from build123d import *

# Parameters (mm, degrees)
F0_W     = 152.4
F0_H     = 50.8
F1_DEPTH = 76.2
F3_DEPTH = 76.201
F5_DEPTH = 152.401


with BuildPart() as f1:
    # F0 (on Front) → F1 (new body)
    with BuildSketch(Plane.XZ):
        with Locations((8.127087, 3.526762)):
            Rectangle(F0_W, F0_H)
    extrude(amount=F1_DEPTH)

    # F2 (on face) → F3 (cut, through all)
    with BuildSketch(Plane.XZ.offset(76.2)):
        Polygon((-40.834155, -12.95126), (-29.972913, -21.873238), (53.436877, -21.873238), (60.765845, -12.95126), align=None)
    extrude(amount=-F3_DEPTH, mode=Mode.SUBTRACT)

    # F4 (on face) → F5 (cut, through all)
    with BuildSketch(Plane.YZ.offset(84.327087)):
        Polygon((-25.4, 28.926762), (-50.8, 28.926762), (-50.8, 16.226762), (-63.5, 16.226762), (-63.5, 3.526762), (-12.7, 3.526762), (-12.7, 16.226762), (-25.4, 16.226762), align=None)
    extrude(amount=-F5_DEPTH, mode=Mode.SUBTRACT)


solid = f1.part
Here's how the part is built. I have some questions about the finished solid (model axes, mm). A direction names the side the tool comes from. Round coordinates to 2 decimals unless told otherwise and drop trailing zeros. Write each loop counter-clockwise with the first axis right and the second up, starting at its lowest first coordinate (ties: lowest second). Pieces come first, ordered by that corner, then holes. Notation, with made-up numbers: (5.5, 19.5) -> (30.5, 19.5) arc R20 cw to (30.5, 27.5) -> close; hole circle Ø8 at (30, -9.75). An arc over 180 degrees is marked (long way). One line per item, written item: value.
1) If I drill on line 1 (Z direction, x = 34.5, y = -20); line 2 (Y direction, x = -54, z = 10.5); line 3 (Y direction, x = -46.5, z = 18.5), over which ranges is the centre line in solid material (lowest first)? Write a range as [from, to].
Filled sheet:
line 1: z = [-12.95, 3.53], [16.23, 28.93]
line 2: y = [-76.2, -63.5], [-12.7, 0]
line 3: y = [-76.2, -50.8], [-25.4, 0]
2) Suppose I cut it at B-B on y = -40.5. List the corners of the cut face in (x, z) for me, plus the area to 3 significant figures.
Filled sheet:
outline: (-68.07, -21.87) -> (-29.97, -21.87) -> (-40.83, -12.95) -> (60.77, -12.95) -> (53.44, -21.87) -> (84.33, -21.87) -> (84.33, 3.53) -> (-68.07, 3.53) -> close
area: 3,050 mm2
3) Suppose I cut it at A-A on z = 24. List the corners of the cut face in (x, y) for me, plus the area to 3 significant figures.
Filled sheet:
outline: (-68.07, -76.2) -> (84.33, -76.2) -> (84.33, -50.8) -> (-68.07, -50.8) -> close; (-68.07, -25.4) -> (84.33, -25.4) -> (84.33, 0) -> (-68.07, 0) -> close
area: 7,740 mm2
4) Suppose I cut it at D-D on z = 11. List the corners of the cut face in (x, y) for me, plus the area to 3 significant figures.
Filled sheet:
outline: (-68.07, -76.2) -> (84.33, -76.2) -> (84.33, -63.5) -> (-68.07, -63.5) -> close; (-68.07, -12.7) -> (84.33, -12.7) -> (84.33, 0) -> (-68.07, 0) -> close
area: 3,870 mm2
5) We'd pull the mould along X, two halves only. Please class faces 1 (the face through (9, -12.7, 10)), 2 (the face through (-35.48, -38.63, -17.35)), 3 (the face through (-68.073, -38, -2)): released by +X, released by -X, zero draft, split by the parting line, or undercut.
Filled sheet:
face 1: zero draft
face 2: undercut
face 3: released by -X
6) Suppose I cut it at C-C on x = 33. List the corners of the cut face in (y, z) for me.
Filled sheet:
outline: (-76.2, -12.95) -> (0, -12.95) -> (0, 28.93) -> (-25.4, 28.93) -> (-25.4, 16.23) -> (-12.7, 16.23) -> (-12.7, 3.53) -> (-63.5, 3.53) -> (-63.5, 16.23) -> (-50.8, 16.23) -> (-50.8, 28.93) -> (-76.2, 28.93) -> close
7) I'm going to push flat-ended pins straight in: pin 1 Ø1.5 at (x, y) = (3, -37.5) entering from -Z; pin 2 Ø15 at (x, y) = (10.5, -42) entering from +Z. Where does each tip first touch, or does it pass through?
Filled sheet:
pin 1: stops at z = -12.95
pin 2: stops at z = 3.53
8) For faces 4 (the face through (9, -19, 16.227)), 5 (the face through (9, -25.4, 22)), 6 (the face through (11, -39, -12.951)), which set-ups out of +Z, -Z, +X, -X, +Y, -Y let a thin tool reach every point of the face, with its end or its side?
Filled sheet:
face 4: +X, -X
face 5: +Z, +X, -X
face 6: +Y, -Y
